Source: CAD feature listing. Evaluate the final solid. Frame: model axes, mm. Coordinates: 2 decimals unless noted, no trailing zeros. Order: outer loops, then holes, each group sorted by start corner. A loop starts at its lowest first (then second) coordinate and runs counter-clockwise, first axis right, second up. Notation, with made-up numbers: (65.25, 54) -> (74.25, 54) arc R24 ccw to (74.25, 85) -> close; hole circle Ø7 at (79, 66.5). An arc over 180 degrees is marked (long way). Put each result on its own line as item: value.
from build123d import *

# Parameters (mm, degrees)
MIEMBRO_ESTRUCTURAL1_DEPTH = 1920


with BuildPart() as part:
    # Sketch1 → Miembro estructural1 (new body)
    with BuildSketch(Plane.YZ.offset(-960)):
        with BuildLine():
            Line((0, 0), (0, 25))
            ThreePointArc((0, 25), (2.828427125, 23.828427125), (4, 21))
            Line((4, 21), (4, 7.5))
            ThreePointArc((4, 7.5), (5.025126266, 5.025126266), (7.5, 4))
            Line((7.5, 4), (21, 4))
            ThreePointArc((21, 4), (23.828427125, 2.828427125), (25, 0))
            Line((25, 0), (0, 0))
        make_face()
    extrude(amount=MIEMBRO_ESTRUCTURAL1_DEPTH)


solid = part.part
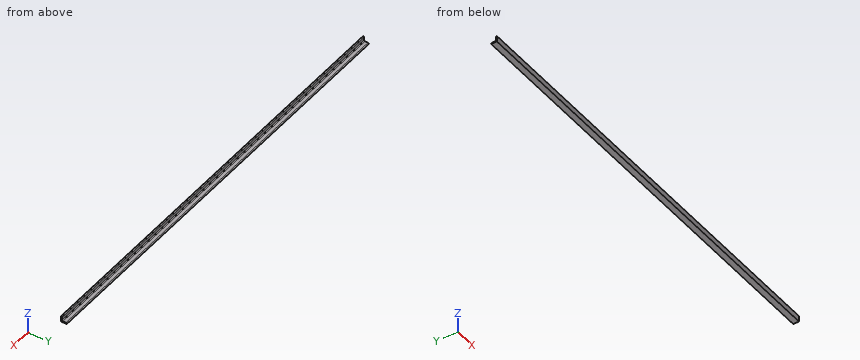
1. Cut plane B-B on y = 12.5. Output: boundary loops of the cut face in (x, z).
Numbers:
outline: (-960, 0) -> (960, 0) -> (960, 4) -> (-960, 4) -> close
2. Ray query, line 1 along Y through (x, z) = (52, 11.75); line 2 along Y through (x, z) = (-570, 1). Return the intervals inside material, ascending.
Numbers:
line 1: y = 0 to 4
line 2: y = 0 to 24.87
3. Cut plane A-A on x = 147. Output: boundary loops of the cut face in (y, z), plus the area to 3 significant figures.
Numbers:
outline: (0, 0) -> (25, 0) arc R4 ccw to (21, 4) -> (7.5, 4) arc R3.5 cw to (4, 7.5) -> (4, 21) arc R4 ccw to (0, 25) -> close
area: 180 mm2
4. First-contact query: pin 1 (15 mm diameter, centred on x = 290.5, y = 15.5, fed in from +Z); pin 2 (12 mm diameter, centred on y = 17, z = 11.5, fed in from +X); pin 3 (7 mm diameter, centred on x = -180, z = 13.5, fed in from +Y). Flat tips, straight axial feed; report the tip coordinate or a pass-through.
Numbers:
pin 1: stops at z = 4
pin 2: passes through
pin 3: stops at y = 4
